Part print with two shaded views. Sizes in mm from the minimum x, y, z corner. A direction names the side the tool comes from. Coordinates: 2 decimals unless noted, no trailing zeros. Write each loop counter-clockwise with the first axis right and the second up, starting at its lowest first coordinate (ties: lowest second). Pieces come first, ordered by that corner, then holes. Notation, with made-up numbers: M 62,-17.5 L 111,-17.5 A18 ccw 111,7.5 Z; hole C 59.5,3 d2. An arc over 180 degrees is marked long. Answer in a Markdown table with one row per item. Add a question column.
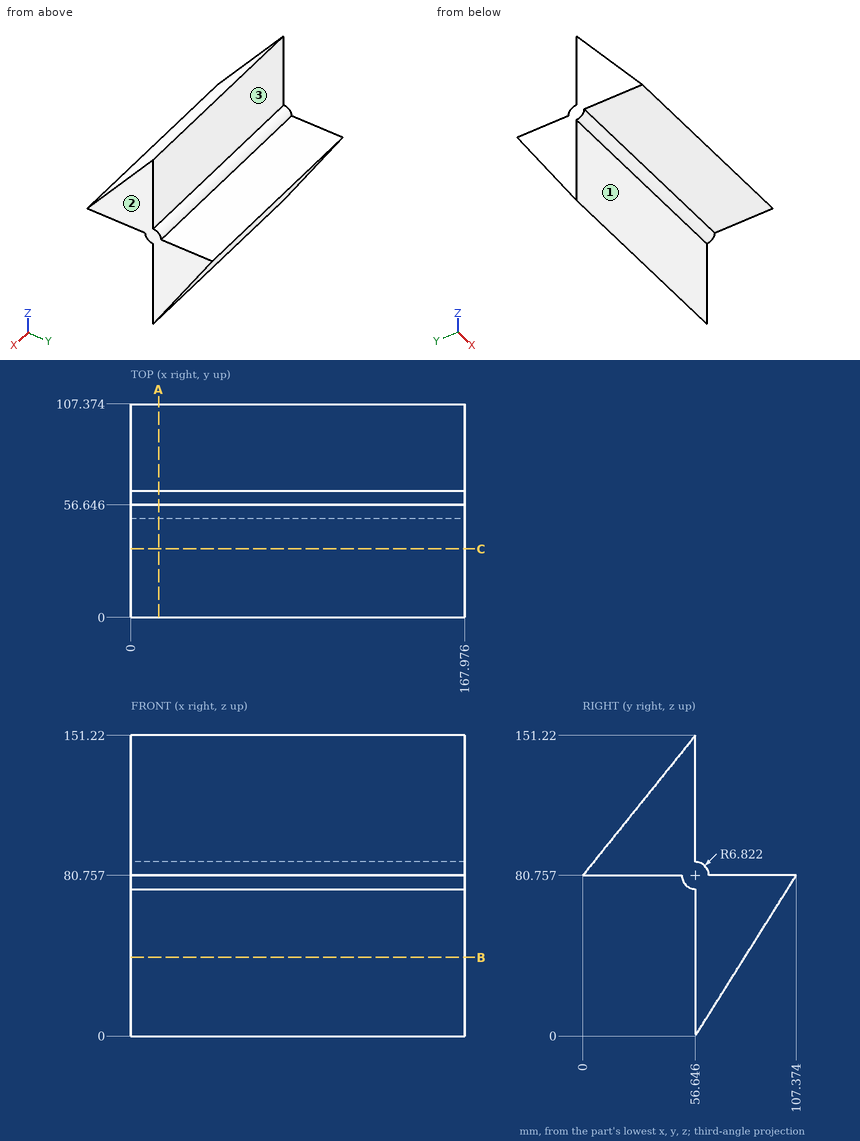
1) Flat gauge pins, fed straight in: pin 1 Ø12 at (y, z) = (95.5, 47.5) entering from +X; pin 2 Ø10 at (x, y) = (79.5, 51.5) entering from -Z; pin 3 Ø19 at (x, z) = (60.5, 130.5) entering from +Y; pin 4 Ø8 at (x, z) = (17, 25.5) entering from +Y. Where does each tip first touch, or does it go through?
2) Slice it at B-B (z = 39.5). Give the cut face in (x, y).
3) Drill centre lines: probe 1 along Y at (x, z) = (159.5, 82) (1 decimal); probe 2 along Y at (x, z) = (10.5, 66.5) (1 decimal); probe 3 along Z at (x, y) = (98, 69.5) (1 decimal). Where is each one in solid material? Low to high.
4) Which spindle directions (+Z, -Z, +X, -X, +Y, -Y) get a long thin tool onto all of the face, cutting with end or side? Do the marked faces 1, 2 and 3. Say none if no direction does.
5) Slice it at C-C (y = 34.5). Give the cut face in (x, z).
6) Slice it at A-A (x = 14). Give the cut face in (y, z) (1 decimal), then the cut area to 3 significant figures.
Ans:
| question | item | result |
|---|---|---|
| 1 | pin 1 | passes through |
| 1 | pin 2 | stops at z = 73.94 |
| 1 | pin 3 | stops at y = 56.65 |
| 1 | pin 4 | stops at y = 75.18 |
| 2 | outline | M 0,56.65 L 167.98,56.65 L 167.98,81.46 L 0,81.46 Z |
| 3 | probe 1 | y = 1 to 63.4 |
| 3 | probe 2 | y = 56.6 to 98.4 |
| 3 | probe 3 | z = 20.5 to 80.8 |
| 4 | face 1 | -Z, +X, -X, -Y |
| 4 | face 2 | +Z, -Z, +X, +Y, -Y |
| 4 | face 3 | +Z, +X, -X, +Y |
| 5 | outline | M 0,80.76 L 167.98,80.76 L 167.98,123.67 L 0,123.67 Z |
| 6 | outline | M 0,80.8 L 49.8,80.8 A6.8 ccw 56.6,73.9 L 56.6,0 L 107.4,80.8 L 63.5,80.8 A6.8 ccw 56.6,87.6 L 56.6,151.2 Z |
| 6 | area | 4,120 mm2 |
